from build123d import *

# Parameters (mm, degrees)
F0_W     = 1400
F0_H     = 650
F1_DEPTH = 25


with BuildPart() as f1:
    # F0 (on Top) → F1 (new body, symmetric)
    with BuildSketch(Plane.XY):
        Polygon((-750, 375), (-750, -375), (-359.724497, -375), (-309.724497, -375), (0, -375), (309.724497, -375), (359.724497, -375), (522.343877, -375), (750, -375), (750, 375), align=None)
        Rectangle(F0_W, F0_H, mode=Mode.SUBTRACT)
    extrude(amount=F1_DEPTH, both=True)


solid = f1.part
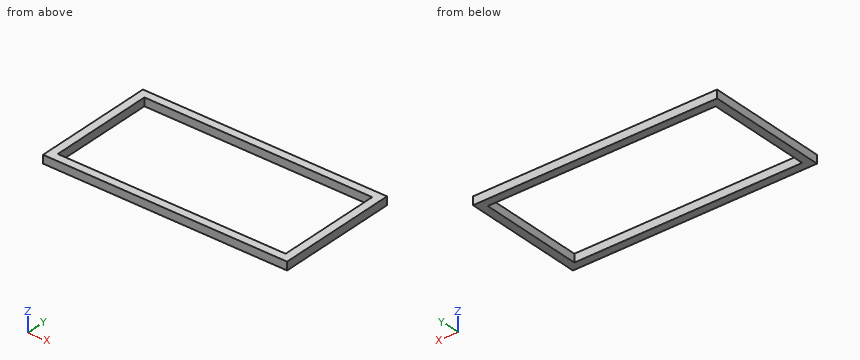
Verification items for the finished model (mm, model axes). Give positions to 0.01 mm unless a question says otherwise; leave off trailing zeros. Write each loop counter-clockwise with the first axis right and the second up, starting at its lowest first coordinate (ties: lowest second). Pieces come first, ordered by that corner, then holes. Notation, with made-up numbers: M 27.5,-18 L 60.5,-18 A15 ccw 60.5,11 Z; hole C 50.5,63.25 d3. An arc over 180 degrees is marked long. Write item = value, one per line.
(1) Sectioned sample at B-B (y = -268.5). Record the cut outline in (x, z).
Found:
outline = M -750,-25 L -700,-25 L -700,25 L -750,25 Z; M 700,-25 L 750,-25 L 750,25 L 700,25 Z
(2) Sectioned sample at C-C (z = 12). Record the cut outline in (x, y).
Found:
outline = M -750,-375 L 750,-375 L 750,375 L -750,375 Z; hole M -700,-325 L 700,-325 L 700,325 L -700,325 Z
(3) Sectioned sample at A-A (x = 499). Record the cut outline in (y, z), then the cut area to 3 significant figures.
Found:
outline = M -375,-25 L -325,-25 L -325,25 L -375,25 Z; M 325,-25 L 375,-25 L 375,25 L 325,25 Z
area = 5,000 mm2
(4) Material ranges on line 1 (X direction, y = 262, z = -5.5); line 2 (Y direction, x = -298, z = 13.5), recorded low to high.
Found:
line_1 = -750 to -700, 700 to 750
line_2 = -375 to -325, 325 to 375
